from build123d import *

# Parameters (mm, degrees)
RESSALTO_EXTRUS_O1_DEPTH = 1.6
ESBO_O2_R                = 1.5
CORTE_EXTRUS_O2_DEPTH    = 2
ESBO_O3_R                = 1.5
CORTE_EXTRUS_O3_DEPTH    = 10
ESBO_O4_R                = 1.5
CORTE_EXTRUS_O4_DEPTH    = 10


with BuildPart() as part:
    # Esboço1 → Ressalto-extrusão1 (new body)
    with BuildSketch(Plane.XY):
        with BuildLine():
            Line((14, 0), (-14, 0))
            Line((-14, 0), (-16, -2))
            Line((-16, -2), (-16, -25))
            Line((-16, -25), (-18, -27))
            Line((-18, -27), (-32, -27))
            Line((-32, -27), (-34, -25))
            Line((-34, -25), (-34, -22))
            Line((-34, -22), (-32, -19))
            Line((-32, -19), (-32, -13))
            Line((-32, -13), (-34, -10))
            Line((-34, -10), (-34, 15))
            Line((-34, 15), (-26, 40))
            Line((-26, 40), (-69.5, 40))
            ThreePointArc((-69.5, 40), (-75.5, 46), (-69.5, 52))
            Line((-69.5, 52), (-20, 52))
            ThreePointArc((-20, 52), (-13.636038969, 54.636038969), (-11, 61))
            Line((-11, 61), (-11, 63))
            Line((-11, 63), (-15, 67))
            Line((-15, 67), (-15, 76))
            Line((-15, 76), (-15.107398643, 76))
            ThreePointArc((-15.107398643, 76), (-23.979715422, 72.299613351), (-32, 67))
            Line((-32, 67), (-46, 67))
            ThreePointArc((-46, 67), (-48.828427125, 68.171572875), (-50, 71))
            ThreePointArc((-50, 71), (0, 92), (50, 71))
            ThreePointArc((50, 71), (48.828427125, 68.171572875), (46, 67))
            Line((46, 67), (32, 67))
            ThreePointArc((32, 67), (23.979715422, 72.299613351), (15.107398643, 76))
            Line((15.107398643, 76), (15, 76))
            Line((15, 76), (15, 67))
            Line((15, 67), (11, 63))
            Line((11, 63), (11, 61))
            ThreePointArc((11, 61), (13.636038969, 54.636038969), (20, 52))
            Line((20, 52), (69.5, 52))
            ThreePointArc((69.5, 52), (75.5, 46), (69.5, 40))
            Line((69.5, 40), (26, 40))
            Line((26, 40), (34, 15))
            Line((34, 15), (34, -10))
            Line((34, -10), (32, -13))
            Line((32, -13), (32, -19))
            Line((32, -19), (34, -22))
            Line((34, -22), (34, -25))
            Line((34, -25), (32, -27))
            Line((32, -27), (18, -27))
            Line((18, -27), (16, -25))
            Line((16, -25), (16, -2))
            Line((16, -2), (14, 0))
        make_face()
    extrude(amount=RESSALTO_EXTRUS_O1_DEPTH)

    # Esboço2 → Corte-extrusão2 (cut)
    with BuildSketch(Plane(origin=(0, 0, 0), x_dir=(-1, 0, 0), z_dir=(0, 0, -1))):
        with Locations((5.5, 66.5)):
            Circle(ESBO_O2_R)
        with Locations((-5.5, 66.5)):
            Circle(ESBO_O2_R)
        with Locations((-5.5, 77.5)):
            Circle(ESBO_O2_R)
        with Locations((5.5, 77.5)):
            Circle(ESBO_O2_R)
        with BuildLine():
            Line((-5, 70), (-9, 70))
            Line((-9, 70), (-9, 74))
            Line((-9, 74), (-5, 74))
            ThreePointArc((-5, 74), (-4.121320344, 76.121320344), (-2, 77))
            Line((-2, 77), (-2, 81))
            Line((-2, 81), (2, 81))
            Line((2, 81), (2, 77))
            ThreePointArc((2, 77), (4.121320344, 76.121320344), (5, 74))
            Line((5, 74), (9, 74))
            Line((9, 74), (9, 70))
            Line((9, 70), (5, 70))
            ThreePointArc((5, 70), (4.121320344, 67.878679656), (2, 67))
            Line((2, 67), (2, 63))
            Line((2, 63), (-2, 63))
            Line((-2, 63), (-2, 67))
            ThreePointArc((-2, 67), (-4.121320344, 67.878679656), (-5, 70))
        make_face()
    extrude(amount=-CORTE_EXTRUS_O2_DEPTH, mode=Mode.SUBTRACT)

    # Esboço3 → Corte-extrusão3 (cut)
    with BuildSketch(Plane.XY.offset(1.6)):
        with Locations((-30.5, -23.5)):
            Circle(ESBO_O3_R)
        with Locations((30.5, -23.5)):
            Circle(ESBO_O3_R)
    extrude(amount=-CORTE_EXTRUS_O3_DEPTH, mode=Mode.SUBTRACT)

    # Esboço4 → Corte-extrusão4 (cut)
    with BuildSketch(Plane.XY.offset(1.6)):
        with Locations((-30.5, -8.5)):
            Circle(ESBO_O4_R)
        with Locations((30.5, -8.5)):
            Circle(ESBO_O4_R)
    extrude(amount=-CORTE_EXTRUS_O4_DEPTH, mode=Mode.SUBTRACT)


solid = part.part
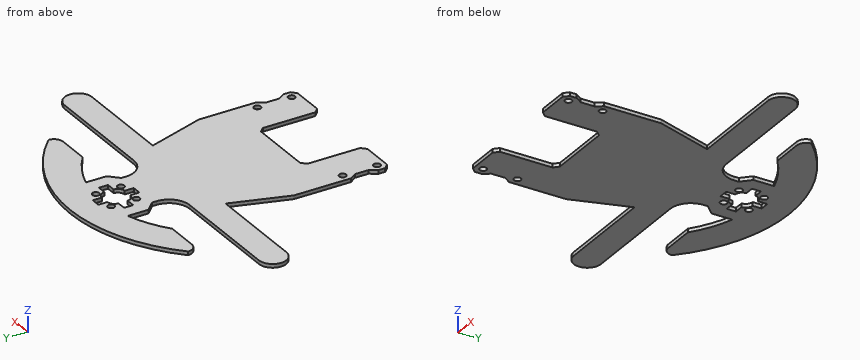
Can you work these out from the model? Positions are in its coordinate system, mm. Round coordinates to 2 decimals unless told otherwise and drop trailing zeros. Loops run counter-clockwise (first coordinate to the right, second up) from the corner with the lowest first, then second, coordinate; pieces in that order, holes last. Notation, with made-up numbers: (29, 49.25) - (36, 49.25) arc R38 cw to (36, 88.25) - close; hole circle Ø7 at (61.25, 49). An arc over 180 degrees is marked (long way). Answer in a Markdown table with one row per item. Add a question column.
Q1. I want a section at B-B on z = 1. Count the separate pieces of the cut face and the enclosed holes in it, and give its area (3 significant figures).
Q2. I want a section at A-A on x = -42.5. List the corners of the cut face in (y, z) for me.
Q3. I want a section at D-D on y = 29.5. List the corners of the cut face in (x, z) for me, and give its area (3 significant figures).
Q4. I want a section at C-C on y = 10. List the corners of the cut face in (x, z) for me, and give its area (3 significant figures).
Q5. I need wall thicknesses on L1, parallel to Y at x = 5.5, z = 0.4; L2, parallel to Y at x = 42.5, z = 0.45; L3, parallel to Y at x = -36.5, z = 0.4. Which ranges of each line are inside material? Lowest first, please.
Q6. For pin 1 Ø0.5 at (x, z) = (-6, 1) entering from +Y; pin 2 Ø0.8 at (y, z) = (72.5, 1) entering from +X; pin 3 Ø0.8 at (y, z) = (78, 1) entering from +X; pin 4 Ø1.8 at (x, y) = (-30.5, -23.5) entering from -Z, each with a flat end and sliding along its axis, tell me the tip position at first contact or that it passes through.
A:
| question | item | result |
|---|---|---|
| 1 | separate pieces | 1 |
| 1 | enclosed holes | 9 |
| 1 | area | 7,070 mm^2 |
| 2 | outline | (40, 0) - (52, 0) - (52, 1.6) - (40, 1.6) - close; (67, 0) - (77.63, 0) - (77.63, 1.6) - (67, 1.6) - close |
| 3 | outline | (-29.36, 0) - (29.36, 0) - (29.36, 1.6) - (-29.36, 1.6) - close |
| 3 | area | 94.0 mm^2 |
| 4 | outline | (-34, 0) - (34, 0) - (34, 1.6) - (-34, 1.6) - close |
| 4 | area | 109 mm^2 |
| 5 | L1 | 0 to 65, 68 to 70, 74 to 76, 79 to 91.78 |
| 5 | L2 | 40 to 52, 67 to 77.63 |
| 5 | L3 | 40 to 52, 67 to 81.73 |
| 6 | pin 1 | y = 91.76 |
| 6 | pin 2 | x = 48.9 |
| 6 | pin 3 | x = 42.54 |
| 6 | pin 4 | through |
